Could you check a few things on this drawing? It's one solid part, dimensions in mm from its lowest x, y, z. Give positions to 0.01 mm unless a question says otherwise; leave off trailing zeros. Order: outer loops, then holes, each group sorted by start corner. A loop starts at its lowest first (then second) coordinate and runs counter-clockwise, first axis right, second up.
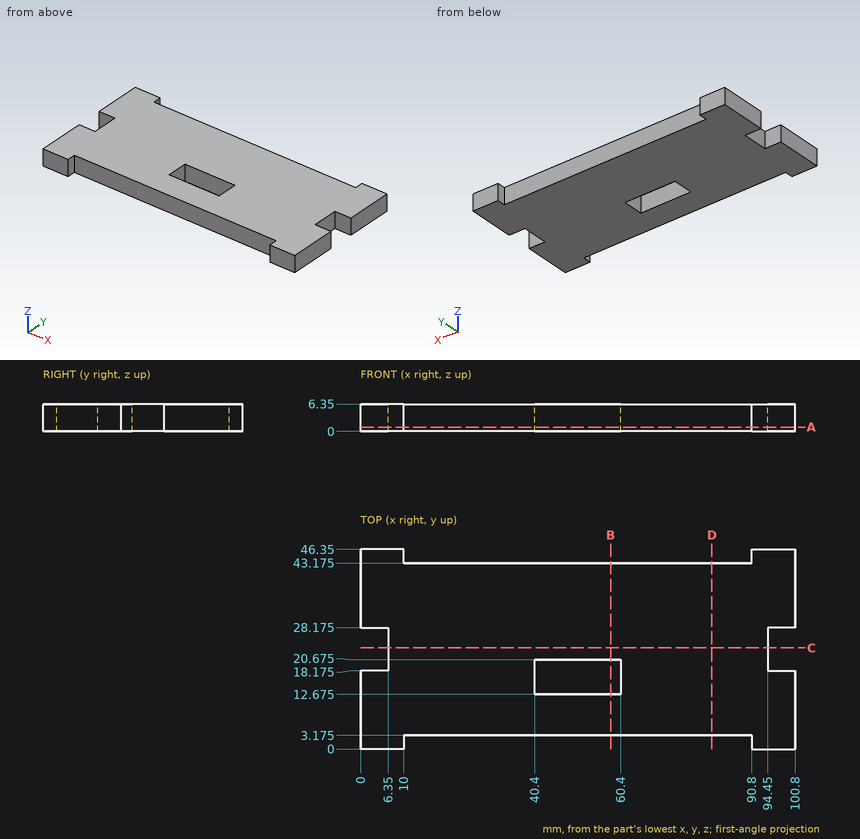
Item 1: Imagine slicing it at C-C on y = 23.5. List the corners of the cut face in (x, z) for me.
Findings:
outline: (6.35, 0) - (94.45, 0) - (94.45, 6.35) - (6.35, 6.35) - close
Item 2: Imagine slicing it at A-A on z = 1. List the corners of the cut face in (x, y) for me (3 decimals), then the cut area to 3 significant figures.
Findings:
outline: (0, 0) - (10, 0) - (10, 3.175) - (90.8, 3.175) - (90.8, 0) - (100.8, 0) - (100.8, 18.175) - (94.45, 18.175) - (94.45, 28.175) - (100.8, 28.175) - (100.8, 46.35) - (90.8, 46.35) - (90.8, 43.175) - (10, 43.175) - (10, 46.35) - (0, 46.35) - (0, 28.175) - (6.35, 28.175) - (6.35, 18.175) - (0, 18.175) - close; hole (40.4, 12.675) - (60.4, 12.675) - (60.4, 20.675) - (40.4, 20.675) - close
area: 3,870 mm2
Item 3: Imagine slicing it at B-B on x = 58. List the corners of the cut face in (y, z) for me (3 decimals), then the cut area to 3 significant figures.
Findings:
outline: (3.175, 0) - (12.675, 0) - (12.675, 6.35) - (3.175, 6.35) - close; (20.675, 0) - (43.175, 0) - (43.175, 6.35) - (20.675, 6.35) - close
area: 203 mm2
Item 4: Please list where these lines run through material, in increasing order: line 1 along X through (y, z) = (14.5, 0.5); line 2 along X through (y, z) = (44.5, 3); line 3 along Y through (x, z) = (57.5, 2.75) (3 decimals).
Findings:
line 1: x = 0 to 40.4, 60.4 to 100.8
line 2: x = 0 to 10, 90.8 to 100.8
line 3: y = 3.175 to 12.675, 20.675 to 43.175
Item 5: For pin 1 (3 mm diameter, centred on x = 39, z = 4, fed in from +Y) (3 decimals); pin 2 (1 mm diameter, centred on y = 44.5, z = 1.5, fed in from -X); pin 3 (1.9 mm diameter, centred on y = 22.5, z = 2, fed in from -X); pin 4 (1.9 mm diameter, centred on y = 23.5, z = 5, fed in from +X), each with a flat end and sliding along its axis, tell me the tip position at first contact or that it passes through.
Findings:
pin 1: stops at y = 43.175
pin 2: stops at x = 0
pin 3: stops at x = 6.35
pin 4: stops at x = 94.45
Item 6: Imagine slicing it at D-D on x = 81.5. List the corners of the cut face in (y, z) for me (3 decimals), then the cut area to 3 significant figures.
Findings:
outline: (3.175, 0) - (43.175, 0) - (43.175, 6.35) - (3.175, 6.35) - close
area: 254 mm2
